```python
from build123d import *

# Parameters (mm, degrees)
F0_R            = 63.5
F1_DEPTH        = 3.175
F3_DEPTH        = 3.175
F3_COPIES_COUNT = 8
F5_DEPTH        = 3.175


# Not quite as in the source:
# - a pattern or mirror of a feature is missing from the dataset's text; its kind, count and spacing are read off the source's solid


with BuildPart() as f1:
    # F0 (on Front) → F1 (new body)
    with BuildSketch(Plane.XZ):
        Circle(F0_R)
    extrude(amount=F1_DEPTH)

    # F2 (on face) → F3 (cut)
    with BuildSketch(Plane.XZ.offset(3.175)):
        with BuildLine():
            Line((0, 63.5), (21.2263563726, 51.2449574344))
            Line((21.2263563726, 51.2449574344), (24.3003979552, 58.6663503145))
            ThreePointArc((24.3003979552, 58.6663503145), (12.388235448, 62.2798653056), (0, 63.5))
        make_face()
    f3 = extrude(amount=-F3_DEPTH, mode=Mode.SUBTRACT)

    # F3_copies: F3 ×8 about axis
    f3_copies_axis = Axis((0, 0, 0), (0, 1, 0))
    for i in range(1, F3_COPIES_COUNT):
        add(f3.rotate(f3_copies_axis, i * 360 / F3_COPIES_COUNT), mode=Mode.SUBTRACT)

    # F4 (on Front) → F5 (cut)
    with BuildSketch(Plane.XZ):
        Polygon((0.1275317148, 12.0983748909), (-10.4137341426, 6.1596331502), (-10.5412658574, -5.9387417407), (-0.1275317148, -12.0983748909), (10.4137341426, -6.1596331502), (10.5412658574, 5.9387417407), align=None)
    extrude(amount=F5_DEPTH, mode=Mode.SUBTRACT)


solid = f1.part
```
Geometry check sheet. Reference: the model listing, model coordinates, mm. A direction names the side the tool comes from. Coordinates: 2 decimals unless noted, no trailing zeros. Loops run counter-clockwise (first coordinate to the right, second up) from the corner with the lowest first, then second, coordinate; pieces in that order, holes last.
Item 1: Go/stop test with flat-tipped pins: pin 1 Ø1.5 at (y, z) = (-1, -19.5) entering from -X; pin 2 Ø1.5 at (y, z) = (-2.5, -45.5) entering from +X. Record where each tip stops, or that it passes through.
Item 2: Access from +Z, -Z, +X, -X, +Y, -Y to the whole of each face (thin tool, end or side, straight path). Record for faces 5 (the face through (22.74, -1.61, -54.9)), 6 (the face through (54.9, -1.61, 22.74)), 7 (the face through (-62.314, -1.565, -12.217)), 8 (the face through (5.407, -1.565, 8.975)).
Item 3: Release check for a two-part mould opening along X. For faces 1 (the face through (-1, -3.175, -13)), 2 (the face through (-54.9, -1.61, 22.74)), 3 (the face through (52.701, -1.565, -35.424)), 4 (the face through (22.74, -1.61, 54.9)) record: released by +X, released by -X, zero draft, split by the parting line, or undercut.
Item 4: Thickness scan on line 1 (Z direction, x = -3.5, y = -0.7); line 2 (Z direction, x = 23, y = -0.6); line 3 (X direction, y = -2.55, z = 29). Record the ranges inside material, lowest first.
Item 5: Sectioned sample at C-C, the plane x = -54.5. Record the boundary of the cut face in (y, z) (3 decimals).
Item 6: Sectioned sample at B-B, the plane x = -7. Record the boundary of the cut face in (y, z) (3 decimals), then the cut area to 3 significant figures.
Item 7: Sectioned sample at D-D, the plane z = -31. Record the boundary of the cut face in (x, y) (3 decimals).
Check result:
1. pin 1: stops at x = -60.67
1. pin 2: stops at x = 45.05
2. face 5: +X, +Y, -Y
2. face 6: +Z, +Y, -Y
2. face 7: -Z, -X, +Y, -Y
2. face 8: +Y, -Y
3. face 1: zero draft
3. face 2: released by -X
3. face 3: released by +X
3. face 4: undercut
4. line 1: z = -61.48 to -10.1, 10.05 to 63.4
4. line 2: z = -59.19 to -55.53, -50.77 to 55.53
4. line 3: x = -56.49 to 49.16
5. outline: (-3.175, -22.575) - (0, -22.575) - (0, 15.588) - (-3.175, 15.588) - close; (-3.175, 22.575) - (0, 22.575) - (0, 32.588) - (-3.175, 32.588) - close
6. outline: (-3.175, -59.459) - (0, -59.459) - (0, -8.033) - (-3.175, -8.033) - close; (-3.175, 8.083) - (0, 8.083) - (0, 63.113) - (-3.175, 63.113) - close
6. area: 338 mm2
7. outline: (-48.626, -3.175) - (55.419, -3.175) - (55.419, 0) - (-48.626, 0) - close
